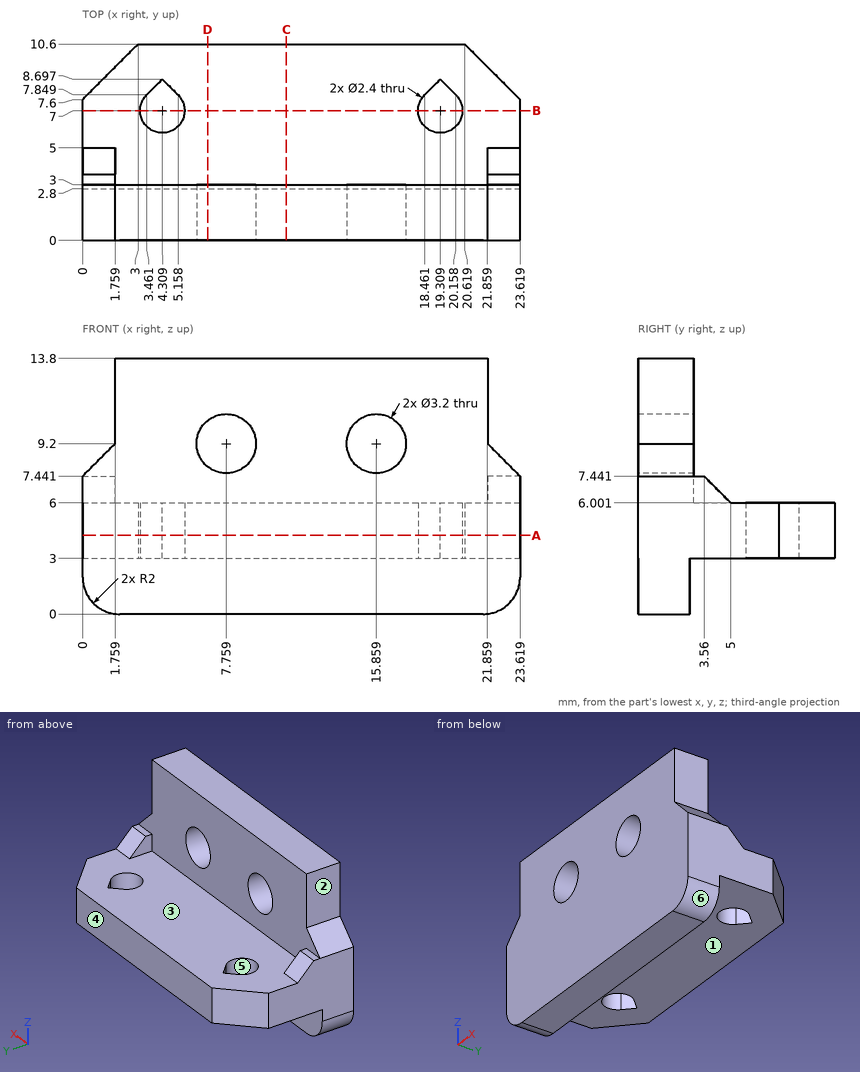
Source: three-view drawing plus pictorial views. Frame: mm from the lowest corner of the part. A direction names the side the tool comes from. Round coordinates to 2 decimals unless told otherwise and drop trailing zeros. Order: outer loops, then holes, each group sorted by start corner. A loop starts at its lowest first (then second) coordinate and runs counter-clockwise, first axis right, second up. Notation, with made-up numbers: (74.25, -9) -> (132.25, -9) arc R19 ccw to (132.25, 19) -> close; hole circle Ø8 at (12.5, 13.5). An arc over 180 degrees is marked (long way). Use one line per item in the form item = value. Start each with the question number.
1. Cut plane D-D (x = 6.75). Return the cut outline in (y, z).
2. Line query: probe 1 along Z at (x, y) = (10, 8.25); probe 2 along Y at (x, z) = (4.5, 2); probe 3 along Y at (x, z) = (21.25, 11). Output: solid intervals per line, ascending.
3. Cut plane B-B (y = 7). Return the cut outline in (x, z).
4. Reachability of the marked faces 1, 2 and 3 from +Z, -Z, +X, -X, +Y, -Y: full face, straight path, thin tool, end or side. Return the list, or none.
5. Draft query along X for the marked faces 4, 5 and 6. Return one class per face: pulls with the +X half, pulls with the -X half, needs draft (parallel to the pull), parting line crosses it, or undercut.
6. Cut plane A-A (z = 4.25). Return the cut outline in (x, y), then the cut area to 3 significant figures.
7. Pin query (flat end, axial travel): pin 1 Ø6 at (x, y) = (6.5, 6) entering from -Z; pin 2 Ø3.5 at (y, z) = (1, 11.5) entering from -X; pin 3 Ø5 at (x, z) = (2.5, 12) entering from -Y; pin 4 Ø3.5 at (x, z) = (15.86, 9.2) entering from +Y. Return the tip coordinate at first contact, or that it passes through.
8. Cut plane C-C (x = 11). Return the cut outline in (y, z).
Solution:
q1.outline = (0, 0) -> (2.8, 0) -> (2.8, 3) -> (10.6, 3) -> (10.6, 6) -> (3, 6) -> (3, 7.96) -> (0, 7.96) -> close; (0, 10.44) -> (3, 10.44) -> (3, 13.8) -> (0, 13.8) -> close
q2.probe_1 = 3 to 6
q2.probe_2 = 0 to 2.8
q2.probe_3 = 0 to 3
q3.outline = (0, 3) -> (3.11, 3) -> (3.11, 6) -> (0, 6) -> close; (5.51, 3) -> (18.11, 3) -> (18.11, 6) -> (5.51, 6) -> close; (20.51, 3) -> (23.62, 3) -> (23.62, 6) -> (20.51, 6) -> close
q4.face_1 = -Z, +X, -X, +Y
q4.face_2 = +Z, -X, +Y, -Y
q4.face_3 = +Z, +Y
q5.face_4 = needs draft
q5.face_5 = undercut
q5.face_6 = pulls with the +X half
q6.outline = (0, 0) -> (23.62, 0) -> (23.62, 7.6) -> (20.62, 10.6) -> (3, 10.6) -> (0, 7.6) -> close; hole (3.46, 7.85) arc R1.2 ccw (long way) to (5.16, 7.85) -> (4.31, 8.7) -> close; hole (18.46, 7.85) arc R1.2 ccw (long way) to (20.16, 7.85) -> (19.31, 8.7) -> close
q6.area = 232 mm^2
q7.pin_1 = 3
q7.pin_2 = 1.76
q7.pin_3 = 0
q7.pin_4 = 3
q8.outline = (0, 0) -> (2.8, 0) -> (2.8, 3) -> (10.6, 3) -> (10.6, 6) -> (3, 6) -> (3, 13.8) -> (0, 13.8) -> close
